Here's how the part is built. I have some questions about the finished solid (model axes, mm). A direction names the side the tool comes from. Round coordinates to 2 decimals unless told otherwise and drop trailing zeros. Loops run counter-clockwise (first coordinate to the right, second up) from the corner with the lowest first, then second, coordinate; pieces in that order, holes last. Notation, with made-up numbers: M -5.75,76.25 L 33.25,76.25 A23 cw 33.25,107.25 Z; hole C -20,40 d9. An arc over 180 degrees is marked long. Use a Markdown table: item, result.
from build123d import *

# Parameters (mm, degrees)
F1_DEPTH = 40
F3_DEPTH = 12.7
F4_DEPTH = 8.89
F6_D     = 3.75
F7_W     = 7
F7_H     = 18.618289
F8_DEPTH = 25.4


with BuildPart() as f1:
    # F0 (on Top) → F1 (new body)
    with BuildSketch(Plane.XY):
        with BuildLine():
            ThreePointArc((-6.452735, 9.21546), (0, 11.25), (6.452735, 9.21546))
            Line((6.452735, 9.21546), (7.599888, 10.853765))
            ThreePointArc((7.599888, 10.853765), (0, 13.25), (-7.599888, 10.853765))
            Line((-7.599888, 10.853765), (-6.452735, 9.21546))
        make_face()
    extrude(amount=F1_DEPTH)

    # F2 (on Top) → F3 (join)
    with BuildSketch(Plane.XY):
        with BuildLine():
            ThreePointArc((-5.25, 9.093267), (0, 10.5), (5.25, 9.093267))
            Line((5.25, 9.093267), (5.625, 9.742786))
            ThreePointArc((5.625, 9.742786), (0, 11.25), (-5.625, 9.742786))
            Line((-5.625, 9.742786), (-5.25, 9.093267))
        make_face()
    extrude(amount=F3_DEPTH)

    # F2 (on Top) → F4 (cut)
    with BuildSketch(Plane.XY):
        with BuildLine():
            ThreePointArc((-5.25, 9.093267), (0, 10.5), (5.25, 9.093267))
            Line((5.25, 9.093267), (5.625, 9.742786))
            ThreePointArc((5.625, 9.742786), (0, 11.25), (-5.625, 9.742786))
            Line((-5.625, 9.742786), (-5.25, 9.093267))
        make_face()
    extrude(amount=F4_DEPTH, mode=Mode.SUBTRACT)

    # F6 (through all)
    with Locations(Plane.XZ):
        with Locations((0, 36), (0, 4)):
            Hole(F6_D / 2)

    # F7 (on Front) → F8 (cut)
    with BuildSketch(Plane.XZ):
        with Locations((0, 22.009144)):
            Rectangle(F7_W, F7_H)
    extrude(amount=-F8_DEPTH, mode=Mode.SUBTRACT)


solid = f1.part
1. Imagine slicing it at A-A, the plane x = 0. Write out the boundary of the cut face in (y, z) (3 decimals), then the cut area to 3 significant figures.
Answer sheet:
| item | result |
|---|---|
| outline | M 10.5,8.89 L 11.25,8.89 L 11.25,5.875 L 13.25,5.875 L 13.25,12.7 L 10.5,12.7 Z; M 11.25,0 L 13.25,0 L 13.25,2.125 L 11.25,2.125 Z; M 11.25,31.318 L 13.25,31.318 L 13.25,34.125 L 11.25,34.125 Z; M 11.25,37.875 L 13.25,37.875 L 13.25,40 L 11.25,40 Z |
| area | 30.6 mm2 |
2. Imagine slicing it at D-D, the plane z = 10.5. Write out the boundary of the cut face in (x, y) (3 decimals), then the cut area to 3 significant figures.
Answer sheet:
| item | result |
|---|---|
| outline | M -7.6,10.854 L -6.453,9.215 A11.25 cw -5.625,9.743 L -5.25,9.093 A10.5 cw 5.25,9.093 L 5.625,9.743 A11.25 cw 6.453,9.215 L 7.6,10.854 A13.25 ccw Z |
| area | 38.5 mm2 |
3. Imagine slicing it at B-B, the plane z = 27. Write out the boundary of the cut face in (x, y), then the cut area to 3 significant figures.
Answer sheet:
| item | result |
|---|---|
| outline | M -7.6,10.85 L -6.45,9.22 A11.25 cw -3.5,10.69 L -3.5,12.78 A13.25 ccw Z; M 3.5,10.69 A11.25 cw 6.45,9.22 L 7.6,10.85 A13.25 ccw 3.5,12.78 Z |
| area | 15.7 mm2 |
4. I need wall thicknesses on probe 1 along Z at (x, y) = (0, 12.05) (3 decimals); probe 2 along Z at (x, y) = (-2, 12.25); probe 3 along X at (y, z) = (11.7, 35). Which ranges of each line are inside material? Lowest first, please. Write a range as from..to.
Answer sheet:
| item | result |
|---|---|
| probe 1 | 0..2.125, 5.875..12.7, 31.318..34.125, 37.875..40 |
| probe 2 | 0..12.7, 31.32..40 |
| probe 3 | -6.22..-1.59, 1.59..6.22 |
5. For pin 1 Ø1.7 at (y, z) = (12, 24.5) entering from -X; pin 2 Ø2 at (x, z) = (-5, 33) entering from +Y; pin 3 Ø1 at (y, z) = (11.5, 26) entering from +X; pin 4 Ø3 at (x, z) = (0, 4) entering from -Y, each with a flat end and sliding along its axis, tell me the tip position at first contact or that it passes through.
Answer sheet:
| item | result |
|---|---|
| pin 1 | x = -7.16 |
| pin 2 | y = 12.63 |
| pin 3 | x = 7.39 |
| pin 4 | through |
6. We'd pull the mould along X, two halves only. Please class faces 1 (the face through (0, 12, 0)), 2 (the face through (7, 10, 20)), 3 (the face through (-7, 10, 20)), 4 (the face through (0, 12, 31.318)): +X half, -X half, draft (parallel to the pull), parting line (faces both ways), or undercut.
Answer sheet:
| item | result |
|---|---|
| face 1 | draft |
| face 2 | +X half |
| face 3 | -X half |
| face 4 | undercut |
7. Imagine slicing it at C-C, the plane x = -3. Write out the boundary of the cut face in (y, z), then the cut area to 3 significant figures.
Answer sheet:
| item | result |
|---|---|
| outline | M 10.06,8.89 L 10.84,8.89 L 10.84,0 L 12.91,0 L 12.91,12.7 L 10.06,12.7 Z; M 10.84,31.32 L 12.91,31.32 L 12.91,40 L 10.84,40 Z |
| area | 47.1 mm2 |
8. Which directions (+Z, -Z, +X, -X, +Y, -Y) give clear straight access to the entire face, cutting with the end or side of a thin tool? Please do faces 5 (the face through (3.662, 12.734, 19.72)), 6 (the face through (0, 11, 8.89)), 7 (the face through (3.5, 12, 22)).
Answer sheet:
| item | result |
|---|---|
| face 5 | +Z, -Z, +Y |
| face 6 | -Z, -Y |
| face 7 | +Y, -Y |
